Read the model definition and answer for the solid it produces. Units are mm, in the model's axes. Face numbers are marked on the shaded views. A direction names the side the tool comes from. Coordinates: 2 decimals unless noted, no trailing zeros. Loops run counter-clockwise (first coordinate to the right, second up) from the corner with the lowest first, then second, coordinate; pieces in that order, holes last.
Q1. The mould has two halves that part along Y. Classify the marked faces 1 and 2: pulls with the +Y half, pulls with the -Y half, needs draft (parallel to the pull), parting line crosses it, or undercut.
Q2. Flat-ended cylindrical pins translate along their axes: P1, Ø4, axis at y = -49, z = 13.5, coming from the +X side; P2, Ø1.5, axis at x = 3.5, y = -10.5, coming from the -Z side; P3, Ø10, axis at x = 3, y = -18, coming from the +Z side; P4, Ø3, axis at y = -17.5, z = 3.5, coming from the -X side. Find the tip coordinate at first contact, or state that the pin passes through.
Q3. Which of the six approach directions +Z, -Z, +X, -X, +Y, -Y give full straight-line access (tool end or side, diameter ignored) to the marked faces 3 and 4?
Q4. Section A-A (y = 0) is taken. Give the vertices of the cut face in (x, z).
Q5. Straight lines are drawn through the part: line 1 (Y direction, x = -6.25, z = 17); line 2 (X direction, y = 43.5, z = 2.25); line 3 (Z direction, x = 5.5, y = 28.5). For each, find the intervals that lie inside material, in ascending order.
Q6. Section D-D (y = 12) is taken. Give the vertices of the cut face in (x, z), then the cut area to 3 significant figures.
Q7. Section B-B (z = 17.75) is taken. Count the separate pieces of the cut face and the enclosed holes in it, then the cut area to 3 significant figures.
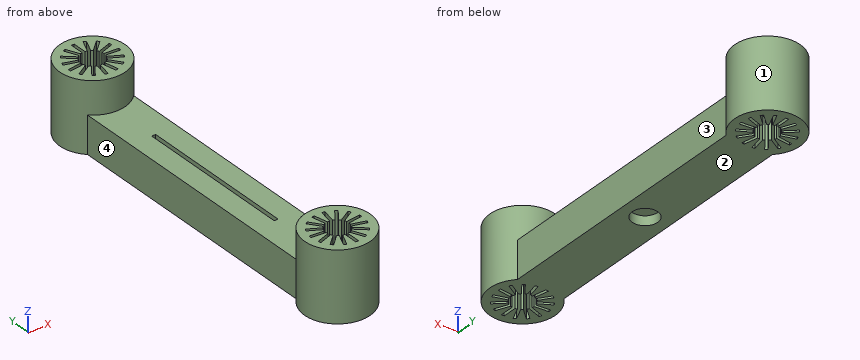
from build123d import *

# Parameters (mm, degrees)
SKETCH1_W                = 12.7
SKETCH1_H                = 86.36
BOSS_EXTRUDE1_DEPTH      = 10.16
SKETCH2_W                = 1.0668
SKETCH2_H                = 43.18
CUT_EXTRUDE1_DEPTH       = 5.08
BOSS_EXTRUDE3_START      = -10.16
SKETCH12_R               = 9
BOSS_EXTRUDE3_DEPTH      = 19.05
SKETCH13_R               = 3.175
CUT_EXTRUDE3_DEPTH       = 57.273038837
SKETCH15_W               = 0.762
SKETCH15_H               = 3.81
CUT_EXTRUDE4_DEPTH       = 57.273038837
CIRPATTERN1_COUNT        = 15
MIRROR2_COPY_1_SKETCH_W  = 0.762
MIRROR2_COPY_1_SKETCH_H  = 3.81
MIRROR2_COPY_1_DEPTH     = 57.273038837
MIRROR2_COPY_2_SKETCH_W  = 0.762
MIRROR2_COPY_2_SKETCH_H  = 3.81
MIRROR2_COPY_2_DEPTH     = 57.273038837
MIRROR2_COPY_3_SKETCH_W  = 0.762
MIRROR2_COPY_3_SKETCH_H  = 3.81
MIRROR2_COPY_3_DEPTH     = 57.273038837
MIRROR2_COPY_4_SKETCH_W  = 0.762
MIRROR2_COPY_4_SKETCH_H  = 3.81
MIRROR2_COPY_4_DEPTH     = 57.273038837
MIRROR2_COPY_5_SKETCH_W  = 0.762
MIRROR2_COPY_5_SKETCH_H  = 3.81
MIRROR2_COPY_5_DEPTH     = 57.273038837
MIRROR2_COPY_6_SKETCH_W  = 0.762
MIRROR2_COPY_6_SKETCH_H  = 3.81
MIRROR2_COPY_6_DEPTH     = 57.273038837
MIRROR2_COPY_7_SKETCH_W  = 0.762
MIRROR2_COPY_7_SKETCH_H  = 3.81
MIRROR2_COPY_7_DEPTH     = 57.273038837
MIRROR2_COPY_8_SKETCH_W  = 0.762
MIRROR2_COPY_8_SKETCH_H  = 3.81
MIRROR2_COPY_8_DEPTH     = 57.273038837
MIRROR2_COPY_9_SKETCH_W  = 0.762
MIRROR2_COPY_9_SKETCH_H  = 3.81
MIRROR2_COPY_9_DEPTH     = 57.273038837
MIRROR2_COPY_10_SKETCH_W = 0.762
MIRROR2_COPY_10_SKETCH_H = 3.81
MIRROR2_COPY_10_DEPTH    = 57.273038837
MIRROR2_COPY_11_SKETCH_W = 0.762
MIRROR2_COPY_11_SKETCH_H = 3.81
MIRROR2_COPY_11_DEPTH    = 57.273038837
MIRROR2_COPY_12_SKETCH_W = 0.762
MIRROR2_COPY_12_SKETCH_H = 3.81
MIRROR2_COPY_12_DEPTH    = 57.273038837
MIRROR2_COPY_13_SKETCH_W = 0.762
MIRROR2_COPY_13_SKETCH_H = 3.81
MIRROR2_COPY_13_DEPTH    = 57.273038837
MIRROR2_COPY_14_SKETCH_W = 0.762
MIRROR2_COPY_14_SKETCH_H = 3.81
MIRROR2_COPY_14_DEPTH    = 57.273038837
M6_CLEARANCE_HOLE1_D     = 7
M6_CLEARANCE_HOLE1_DEPTH = 2.54


with BuildPart() as part:
    # Sketch1 → Boss-Extrude1 (new body)
    with BuildSketch(Plane.XY):
        Rectangle(SKETCH1_W, SKETCH1_H)
    extrude(amount=BOSS_EXTRUDE1_DEPTH)

    # Sketch2 → Cut-Extrude1 (cut)
    with BuildSketch(Plane.XY.offset(10.16)):
        with Locations((-0.0254, 0)):
            Rectangle(SKETCH2_W, SKETCH2_H)
    extrude(amount=-CUT_EXTRUDE1_DEPTH, mode=Mode.SUBTRACT)

    # Sketch12 → Boss-Extrude3 (add)
    with BuildSketch(Plane.XY.offset(10.16).offset(BOSS_EXTRUDE3_START)):
        with Locations((0, 43.18)):
            Circle(SKETCH12_R)
    boss_extrude3 = extrude(amount=BOSS_EXTRUDE3_DEPTH)

    # Sketch13 → Cut-Extrude3 (cut, through all)
    with BuildSketch(Plane.XY.offset(19.05)):
        with Locations((0, 43.18)):
            Circle(SKETCH13_R)
    cut_extrude3 = extrude(amount=-CUT_EXTRUDE3_DEPTH, mode=Mode.SUBTRACT)

    # Sketch15 → Cut-Extrude4 (cut, through all)
    with BuildSketch(Plane.XY.offset(19.05)):
        with Locations((0, 48.237057106)):
            Rectangle(SKETCH15_W, SKETCH15_H)
    cut_extrude4 = extrude(amount=-CUT_EXTRUDE4_DEPTH, mode=Mode.SUBTRACT)

    # CirPattern1: Cut-Extrude4 ×15 about axis
    cirpattern1_axis = Axis((0, 43.18, 0), (0, 0, 1))
    for i in range(1, CIRPATTERN1_COUNT):
        add(cut_extrude4.rotate(cirpattern1_axis, i * 360 / CIRPATTERN1_COUNT), mode=Mode.SUBTRACT)

    # Mirror2: Boss-Extrude3, Cut-Extrude3, Cut-Extrude4 across plane
    add(boss_extrude3.mirror(Plane.ZX))
    add(cut_extrude3.mirror(Plane.ZX), mode=Mode.SUBTRACT)
    add(cut_extrude4.mirror(Plane.ZX), mode=Mode.SUBTRACT)

    # Mirror2 copy 1 sketch → Mirror2 copy 1 (cut, through all)
    with BuildSketch(Plane(origin=(17.562888248, -3.733107139, 19.05), x_dir=(0.9135454576426009, -0.4067366430758002, 0), z_dir=(0, 0, 1))):
        with Locations((0, -48.237057106)):
            Rectangle(MIRROR2_COPY_1_SKETCH_W, MIRROR2_COPY_1_SKETCH_H)
    extrude(amount=-MIRROR2_COPY_1_DEPTH, mode=Mode.SUBTRACT)

    # Mirror2 copy 2 sketch → Mirror2 copy 2 (cut, through all)
    with BuildSketch(Plane(origin=(32.088993564, -14.286940417, 19.05), x_dir=(0.6691306063588582, -0.7431448254773942, 0), z_dir=(0, 0, 1))):
        with Locations((0, -48.237057106)):
            Rectangle(MIRROR2_COPY_2_SKETCH_W, MIRROR2_COPY_2_SKETCH_H)
    extrude(amount=-MIRROR2_COPY_2_DEPTH, mode=Mode.SUBTRACT)

    # Mirror2 copy 3 sketch → Mirror2 copy 3 (cut, through all)
    with BuildSketch(Plane(origin=(41.066620374, -29.836646183, 19.05), x_dir=(0.30901699437494745, -0.9510565162951535, 0), z_dir=(0, 0, 1))):
        with Locations((0, -48.237057106)):
            Rectangle(MIRROR2_COPY_3_SKETCH_W, MIRROR2_COPY_3_SKETCH_H)
    extrude(amount=-MIRROR2_COPY_3_DEPTH, mode=Mode.SUBTRACT)

    # Mirror2 copy 4 sketch → Mirror2 copy 4 (cut, through all)
    with BuildSketch(Plane(origin=(42.943455442, -47.693539044, 19.05), x_dir=(-0.10452846326765355, -0.9945218953682733, 0), z_dir=(0, 0, 1))):
        with Locations((0, -48.237057106)):
            Rectangle(MIRROR2_COPY_4_SKETCH_W, MIRROR2_COPY_4_SKETCH_H)
    extrude(amount=-MIRROR2_COPY_4_DEPTH, mode=Mode.SUBTRACT)

    # Mirror2 copy 5 sketch → Mirror2 copy 5 (cut, through all)
    with BuildSketch(Plane(origin=(37.394976935, -64.77, 19.05), x_dir=(-0.4999999999999998, -0.8660254037844387, 0), z_dir=(0, 0, 1))):
        with Locations((0, -48.237057106)):
            Rectangle(MIRROR2_COPY_5_SKETCH_W, MIRROR2_COPY_5_SKETCH_H)
    extrude(amount=-MIRROR2_COPY_5_DEPTH, mode=Mode.SUBTRACT)

    # Mirror2 copy 6 sketch → Mirror2 copy 6 (cut, through all)
    with BuildSketch(Plane(origin=(25.380567194, -78.113353817, 19.05), x_dir=(-0.8090169943749473, -0.5877852522924732, 0), z_dir=(0, 0, 1))):
        with Locations((0, -48.237057106)):
            Rectangle(MIRROR2_COPY_6_SKETCH_W, MIRROR2_COPY_6_SKETCH_H)
    extrude(amount=-MIRROR2_COPY_6_DEPTH, mode=Mode.SUBTRACT)

    # Mirror2 copy 7 sketch → Mirror2 copy 7 (cut, through all)
    with BuildSketch(Plane(origin=(8.97762681, -85.4164134, 19.05), x_dir=(-0.9781476007338057, -0.20791169081775931, 0), z_dir=(0, 0, 1))):
        with Locations((0, -48.237057106)):
            Rectangle(MIRROR2_COPY_7_SKETCH_W, MIRROR2_COPY_7_SKETCH_H)
    extrude(amount=-MIRROR2_COPY_7_DEPTH, mode=Mode.SUBTRACT)

    # Mirror2 copy 8 sketch → Mirror2 copy 8 (cut, through all)
    with BuildSketch(Plane(origin=(-8.97762681, -85.4164134, 19.05), x_dir=(-0.9781476007338056, 0.2079116908177595, 0), z_dir=(0, 0, 1))):
        with Locations((0, -48.237057106)):
            Rectangle(MIRROR2_COPY_8_SKETCH_W, MIRROR2_COPY_8_SKETCH_H)
    extrude(amount=-MIRROR2_COPY_8_DEPTH, mode=Mode.SUBTRACT)

    # Mirror2 copy 9 sketch → Mirror2 copy 9 (cut, through all)
    with BuildSketch(Plane(origin=(-25.380567194, -78.113353817, 19.05), x_dir=(-0.8090169943749476, 0.587785252292473, 0), z_dir=(0, 0, 1))):
        with Locations((0, -48.237057106)):
            Rectangle(MIRROR2_COPY_9_SKETCH_W, MIRROR2_COPY_9_SKETCH_H)
    extrude(amount=-MIRROR2_COPY_9_DEPTH, mode=Mode.SUBTRACT)

    # Mirror2 copy 10 sketch → Mirror2 copy 10 (cut, through all)
    with BuildSketch(Plane(origin=(-37.394976935, -64.77, 19.05), x_dir=(-0.5000000000000004, 0.8660254037844384, 0), z_dir=(0, 0, 1))):
        with Locations((0, -48.237057106)):
            Rectangle(MIRROR2_COPY_10_SKETCH_W, MIRROR2_COPY_10_SKETCH_H)
    extrude(amount=-MIRROR2_COPY_10_DEPTH, mode=Mode.SUBTRACT)

    # Mirror2 copy 11 sketch → Mirror2 copy 11 (cut, through all)
    with BuildSketch(Plane(origin=(-42.943455442, -47.693539044, 19.05), x_dir=(-0.10452846326765336, 0.9945218953682734, 0), z_dir=(0, 0, 1))):
        with Locations((0, -48.237057106)):
            Rectangle(MIRROR2_COPY_11_SKETCH_W, MIRROR2_COPY_11_SKETCH_H)
    extrude(amount=-MIRROR2_COPY_11_DEPTH, mode=Mode.SUBTRACT)

    # Mirror2 copy 12 sketch → Mirror2 copy 12 (cut, through all)
    with BuildSketch(Plane(origin=(-41.066620374, -29.836646183, 19.05), x_dir=(0.30901699437494723, 0.9510565162951536, 0), z_dir=(0, 0, 1))):
        with Locations((0, -48.237057106)):
            Rectangle(MIRROR2_COPY_12_SKETCH_W, MIRROR2_COPY_12_SKETCH_H)
    extrude(amount=-MIRROR2_COPY_12_DEPTH, mode=Mode.SUBTRACT)

    # Mirror2 copy 13 sketch → Mirror2 copy 13 (cut, through all)
    with BuildSketch(Plane(origin=(-32.088993564, -14.286940417, 19.05), x_dir=(0.6691306063588578, 0.7431448254773946, 0), z_dir=(0, 0, 1))):
        with Locations((0, -48.237057106)):
            Rectangle(MIRROR2_COPY_13_SKETCH_W, MIRROR2_COPY_13_SKETCH_H)
    extrude(amount=-MIRROR2_COPY_13_DEPTH, mode=Mode.SUBTRACT)

    # Mirror2 copy 14 sketch → Mirror2 copy 14 (cut, through all)
    with BuildSketch(Plane(origin=(-17.562888248, -3.733107139, 19.05), x_dir=(0.913545457642601, 0.40673664307580015, 0), z_dir=(0, 0, 1))):
        with Locations((0, -48.237057106)):
            Rectangle(MIRROR2_COPY_14_SKETCH_W, MIRROR2_COPY_14_SKETCH_H)
    extrude(amount=-MIRROR2_COPY_14_DEPTH, mode=Mode.SUBTRACT)

    # M6 Clearance Hole1
    with Locations(Plane(origin=(0, 0, 0), x_dir=(-1, 0, 0), z_dir=(0, 0, -1))):
        with Locations((0, 0)):
            Hole(M6_CLEARANCE_HOLE1_D / 2, depth=M6_CLEARANCE_HOLE1_DEPTH)


solid = part.part
Numbers:
1. face 1: undercut
1. face 2: needs draft
2. P1: stops at x = 8.15
2. P2: stops at z = 0
2. P3: stops at z = 10.16
2. P4: stops at x = -6.35
3. face 3: +Z, -Z, +X
3. face 4: +Z, -Z, -X
4. outline: (-6.35, 0) - (-3.5, 0) - (-3.5, 2.54) - (3.5, 2.54) - (3.5, 0) - (6.35, 0) - (6.35, 10.16) - (0.51, 10.16) - (0.51, 5.08) - (-0.56, 5.08) - (-0.56, 10.16) - (-6.35, 10.16) - close
5. line 1: y = -49.66 to -45.61, -44.81 to -42.91, -42.14 to -36.7, 36.7 to 42.14, 42.91 to 44.81, 45.61 to 49.66
5. line 2: x = -8.99 to -3.16, 3.16 to 8.99
5. line 3: z = 0 to 10.16
6. outline: (-6.35, 0) - (6.35, 0) - (6.35, 10.16) - (0.51, 10.16) - (0.51, 5.08) - (-0.56, 5.08) - (-0.56, 10.16) - (-6.35, 10.16) - close
6. area: 124 mm2
7. separate pieces: 2
7. enclosed holes: 2
7. area: 359 mm2
